Part model, mm, in its own coordinate system. A direction names the side the tool comes from. Coordinates: 2 decimals unless noted, no trailing zeros. Write each loop counter-clockwise with the first axis right and the second up, starting at its lowest first coordinate (ties: lowest second). Pieces come first, ordered by that corner, then holes. Notation, with made-up numbers: M 8.5,-25.75 L 21.5,-25.75 A31 cw 21.5,0.25 Z; hole C 19.5,-38.75 d2. An arc over 180 degrees is marked long. Use a Markdown table: item, result. Add a question column.
Q1. Slice it at A-A on z = 4. Write the cut outline in (x, y), then the cut area to 3 significant figures.
Q2. Wall check: L1, parallel to Y at x = -27, z = 1; L2, parallel to X at y = -27.5, z = 3.25; L3, parallel to Z at x = 11.5, y = -38.5. Give the ranges that are in metal, low to high. Write a range as from..to.
Q3. Slice it at D-D on y = -20.5. Write the cut outline in (x, z).
Q4. Slice it at B-B on y = -81.5. Write the cut outline in (x, z), then the cut area to 3 significant figures.
Q5. Mould opens along Y. For faces 4 (the cylindrical face through (17.6, -89.6, 0.7)), 5 (the cylindrical face through (-80.4, -89.6, 0.7)), 6 (the flat face through (-68, -13, 9.5)), 7 (the flat face through (-68, -7.857, 5)) say: released by +Y, released by -Y, zero draft, split by the parting line, or undercut.
Q6. Pin check, flat tips, straight feed: pin 1 Ø3 at (y, z) = (-27, 6) entering from -X; pin 2 Ø1 at (x, z) = (-41, 10.5) entering from +Y; pin 3 Ø1 at (y, z) = (-52, 10) entering from +X. Stop position of each tip, or through.
Q7. Tool access for faces 1 (the flat face through (6, -13, 9.5)), 2 (the flat face through (4.519, -28, 5)), 3 (the flat face through (3, -47.857, 10)): list every direction of +Z, -Z, +X, -X, +Y, -Y with a clear straight run to the whole face (end or side of a thin tool).
Q8. Slice it at C-C on x = -28.5. Write the cut outline in (y, z).
from build123d import *

# Parameters (mm, degrees)
SKETCH_1_R           = 2
EXTRUDE_1_DEPTH      = 1.5
SKETCH_2_W           = 3
SKETCH_2_H           = 50
SKETCH_2_H_2         = 40
EXTRUDE_3_DEPTH      = 8
EXTRUDE_4_DEPTH      = 2
SKETCH_4_W           = 71.000000198
SKETCH_4_H           = 50
CUT_EXTRUDE_1_DEPTH  = 128.300477144
CUT_EXTRUDE_3_DEPTH  = 128.427082997
HOLE_WIZARD_M2_5_1_D = 2.55
SKETCH_11_W          = 18.075
SKETCH_11_H          = 14.197672296
CUT_EXTRUDE_4_DEPTH  = 128.300477144


with BuildPart() as part:
    # 草圖1 → 填料-伸長1 (new body)
    with BuildSketch(Plane.XY):
        with BuildLine():
            Line((-78.58357781, -93.341907955), (16.519190028, -93.341907955))
            Line((16.519190028, -93.341907955), (23.019189929, -93.341907955))
            ThreePointArc((23.019189929, -93.341907955), (23.72629671, -93.049014736), (24.019189929, -92.341907955))
            Line((24.019189929, -92.341907955), (24.019189929, -26.916101175))
            ThreePointArc((24.019189929, -26.916101175), (23.715868617, -26.228364762), (23.019189929, -25.946187519))
            Line((23.019189929, -25.946187519), (16.519190028, -25.946187519))
            ThreePointArc((16.519190028, -25.946187519), (11.569442559, -23.895934988), (9.519190028, -18.946187519))
            Line((9.519190028, -18.946187519), (9.519190028, -5.659090909))
            ThreePointArc((9.519190028, -5.659090909), (9.226296809, -4.951984128), (8.519190028, -4.659090909))
            Line((8.519190028, -4.659090909), (-70.48081017, -4.659090909))
            ThreePointArc((-70.48081017, -4.659090909), (-71.187916951, -4.951984128), (-71.48081017, -5.659090909))
            Line((-71.48081017, -5.659090909), (-71.48081017, -18.946187519))
            ThreePointArc((-71.48081017, -18.946187519), (-73.531062702, -23.895934988), (-78.48081017, -25.946187519))
            Line((-78.48081017, -25.946187519), (-84.980810071, -25.946187519))
            ThreePointArc((-84.980810071, -25.946187519), (-85.687916853, -26.239080738), (-85.980810071, -26.946187519))
            Line((-85.980810071, -26.946187519), (-85.980810071, -92.341911374))
            ThreePointArc((-85.980810071, -92.341911374), (-85.688840793, -93.048093006), (-84.983425077, -93.341907955))
            Line((-84.983425077, -93.341907955), (-78.58357781, -93.341907955))
        make_face()
        with Locations((-79.980810071, -31.644049447)):
            Circle(SKETCH_1_R, mode=Mode.SUBTRACT)
        with Locations((18.019189929, -31.644049447)):
            Circle(SKETCH_1_R, mode=Mode.SUBTRACT)
        with Locations((18.019189929, -87.644049447)):
            Circle(SKETCH_1_R, mode=Mode.SUBTRACT)
        with Locations((-79.980810071, -87.644049447)):
            Circle(SKETCH_1_R, mode=Mode.SUBTRACT)
    extrude(amount=EXTRUDE_1_DEPTH)

    # 草圖2 → 填料-伸長3 (add)
    with BuildSketch(Plane.XY.offset(1.5)):
        with Locations((-67.98081017, -32.85713984)):
            Rectangle(SKETCH_2_W, SKETCH_2_H)
        with Locations((6.019190028, -27.85713984)):
            Rectangle(SKETCH_2_W, SKETCH_2_H_2)
    extrude(amount=EXTRUDE_3_DEPTH)

    # 草圖3 → 填料-伸長4 (add)
    with BuildSketch(Plane.XY.offset(9.5)):
        Polygon((-69.48081017, -17.828011501), (7.519190028, -17.828011501), (7.519190028, -47.85713984), (-8.225095928, -47.85713984), (-8.225095928, -57.85713984), (-69.48081017, -57.85713984), align=None)
    extrude(amount=EXTRUDE_4_DEPTH)

    # 草圖4 → 除料-伸長1 (cut, through all)
    with BuildSketch(Plane.XY.offset(1.5)):
        with Locations((-30.980810071, -32.85713984)):
            Rectangle(SKETCH_4_W, SKETCH_4_H)
    extrude(amount=-CUT_EXTRUDE_1_DEPTH, mode=Mode.SUBTRACT)

    # 草圖7 → 除料-伸長3 (cut, through all)
    with BuildSketch(Plane.XY.offset(11.5)):
        Polygon((-16.225095928, -49.85713984), (-16.225095928, -39.85713984), (-0.480809972, -39.85713984), (-0.480809972, -25.828011501), (-61.48081017, -25.828011501), (-61.48081017, -49.85713984), align=None)
    extrude(amount=-CUT_EXTRUDE_3_DEPTH, mode=Mode.SUBTRACT)

    # M2.5 螺旋的螺孔鑽1 (through all)
    with Locations(Plane.XY.offset(1.5)):
        with Locations((10.589404461, -68.244235659), (-5.010595539, -68.244235659), (-10.419668394, -72.571170345), (-38.419668394, -72.571170345), (-42.919668394, -69.961668418), (-70.919668394, -69.961668418)):
            Hole(HOLE_WIZARD_M2_5_1_D / 2)

    # 草圖11 → 除料-伸長4 (cut, through all)
    with BuildSketch(Plane.XY.offset(1.5)):
        with Locations((2.751904461, -86.243071807)):
            Rectangle(SKETCH_11_W, SKETCH_11_H)
    extrude(amount=-CUT_EXTRUDE_4_DEPTH, mode=Mode.SUBTRACT)


solid = part.part
Recorded:
| question | item | result |
|---|---|---|
| 1 | outline | M -69.48,-57.86 L -66.48,-57.86 L -66.48,-7.86 L -69.48,-7.86 Z; M 4.52,-47.86 L 7.52,-47.86 L 7.52,-7.86 L 4.52,-7.86 Z |
| 1 | area | 270 mm² |
| 2 | L1 | -93.34..-57.86, -7.86..-4.66 |
| 2 | L2 | -69.48..-66.48, 4.52..7.52 |
| 2 | L3 | 0..1.5 |
| 3 | outline | M -71.66,0 L -66.48,0 L -66.48,9.5 L 4.52,9.5 L 4.52,0 L 9.69,0 L 9.69,1.5 L 7.52,1.5 L 7.52,11.5 L -69.48,11.5 L -69.48,1.5 L -71.66,1.5 Z |
| 4 | outline | M -85.98,0 L -6.29,0 L -6.29,1.5 L -85.98,1.5 Z; M 11.79,0 L 24.02,0 L 24.02,1.5 L 11.79,1.5 Z |
| 4 | area | 138 mm² |
| 5 | face 4 | undercut |
| 5 | face 5 | undercut |
| 5 | face 6 | zero draft |
| 5 | face 7 | released by +Y |
| 6 | pin 1 | x = -69.48 |
| 6 | pin 2 | y = -17.83 |
| 6 | pin 3 | x = -8.23 |
| 7 | face 1 | +Z, +X, -X, +Y |
| 7 | face 2 | -Z |
| 7 | face 3 | +Z, +X, -Y |
| 8 | outline | M -93.34,0 L -57.86,0 L -57.86,1.5 L -93.34,1.5 Z; M -57.86,9.5 L -49.86,9.5 L -49.86,11.5 L -57.86,11.5 Z; M -25.83,9.5 L -17.83,9.5 L -17.83,11.5 L -25.83,11.5 Z; M -7.86,0 L -4.66,0 L -4.66,1.5 L -7.86,1.5 Z |
